Build history of the part. All positions in model axes, mm. A direction names the side the tool comes from. Round coordinates to 2 decimals unless told otherwise and drop trailing zeros. Write each loop counter-clockwise with the first axis right and the second up, starting at its lowest first coordinate (ties: lowest second). Pieces come first, ordered by that corner, then holes.
1) Saw through at A-A (z = 0). Write the cut outline in (x, y).
2) Saw through at B-B (x = 0). Write the cut outline in (y, z), plus the area to 3 significant figures.
3) Saw through at C-C (y = 11.25). Write the cut outline in (x, z).
4) Wall check: probe 1 along X at (y, z) = (25.75, -10.5); probe 2 along X at (y, z) = (26.05, 0); probe 3 along X at (y, z) = (13.75, -4). Give the ranges that are in metal, low to high.
5) Pull direction Z, two halves, no side cores. Call faces 3 (the cylindrical face through (24.986, 0.301, -14.715)), 4 (the cylindrical face through (-24.99, 14.58, 0.27)), 5 (the flat face through (24, 12, 0)): +Z half, -Z half, draft (parallel to the pull), parting line (faces both ways), or undercut.
6) Saw through at D-D (x = 20). Write the cut outline in (y, z), plus the area to 3 significant figures.
7) Which spindle directions (+Z, -Z, +X, -X, +Y, -Y) get a long thin tool onto all of the face, cutting with end or side? Do faces 1 (the cylindrical face through (24.986, 0.285, 6.501)), 2 (the flat face through (0, 26.8, 7)). Say none if no direction does.
8) Flat gauge pin, fed straight in: pin 1 (8 mm diameter, centred on x = 7.5, z = -9, fed in from -Y). Where does the tip first touch, or does it go through?
from build123d import *

# Parameters (mm, degrees)
BOSS_EXTRU_1_DEPTH      = 15
ESQUISSE4_R             = 6.25
ESQUISSE4_R_2           = 1.55
ENL_V_MAT_EXTRU_2_DEPTH = 41.239781312
ESQUISSE2_R             = 1.25
ENL_V_MAT_EXTRU_1_DEPTH = 61.392383626
CONG_1_R                = 1


with BuildPart() as part:
    # Esquisse1 → Boss.-Extru.1 (new, symmetric)
    with BuildSketch(Plane.XY):
        Polygon((-26, 26.8), (26, 26.8), (26, 0), (24, 0), (24, 24.8), (-24, 24.8), (-24, 0), (-26, 0), align=None)
    extrude(amount=BOSS_EXTRU_1_DEPTH, both=True)

    # Esquisse4 → Enlèv. mat.-Extru.2 (cut, through all)
    with BuildSketch(Plane(origin=(0, 26.8, 0), x_dir=(1, 0, 0), z_dir=(0, 1, 0))):
        with Locations(Location((0, 0, 0), (0, 0, 270))):
            Circle(ESQUISSE4_R)
        with Locations(Location((-8.485281374, 8.485281374, 0), (0, 0, 270))):
            Circle(ESQUISSE4_R_2)
        with Locations(Location((8.485281374, 8.485281374, 0), (0, 0, 270))):
            Circle(ESQUISSE4_R_2)
        with Locations(Location((8.485281374, -8.485281374, 0), (0, 0, 270))):
            Circle(ESQUISSE4_R_2)
        with Locations(Location((-8.485281374, -8.485281374, 0), (0, 0, 270))):
            Circle(ESQUISSE4_R_2)
        with Locations(Location((20, 10.5, 0), (0, 0, 270))):
            Circle(ESQUISSE4_R_2)
        with Locations(Location((-20, 10.5, 0), (0, 0, 270))):
            Circle(ESQUISSE4_R_2)
        with Locations(Location((20, -10.5, 0), (0, 0, 270))):
            Circle(ESQUISSE4_R_2)
        with Locations(Location((-20, -10.5, 0), (0, 0, 270))):
            Circle(ESQUISSE4_R_2)
    extrude(amount=-ENL_V_MAT_EXTRU_2_DEPTH, mode=Mode.SUBTRACT)

    # Esquisse2 → Enlèv. mat.-Extru.1 (cut, through all)
    with BuildSketch(Plane(origin=(26, 0, 0), x_dir=(0, 0, -1), z_dir=(1, 0, 0))):
        with Locations((-12, 15.8)):
            Circle(ESQUISSE2_R)
        with Locations((-12, 3.8)):
            Circle(ESQUISSE2_R)
        with Locations((0, 15.8)):
            Circle(ESQUISSE2_R)
        with Locations((12, 3.8)):
            Circle(ESQUISSE2_R)
        with Locations((12, 15.8)):
            Circle(ESQUISSE2_R)
        with BuildLine():
            Line((-6.2, 3.8), (-6.2, 0))
            Line((-6.2, 0), (6.2, 0))
            Line((6.2, 0), (6.2, 3.8))
            ThreePointArc((6.2, 3.8), (0, 10), (-6.2, 3.8))
        make_face()
    extrude(amount=-ENL_V_MAT_EXTRU_1_DEPTH, mode=Mode.SUBTRACT)

    # Congé1
    cong_1_edges = [part.edges().sort_by_distance(p)[0] for p in [
        (-25, 0, -6.2),
        (25, 0, -6.2),
        (-25, 0, 6.2),
        (25, 0, 6.2),
        (25, 0, 15),
        (-25, 0, 15),
        (-25, 0, -15),
        (25, 0, -15),
    ]]
    fillet(cong_1_edges, radius=CONG_1_R)


solid = part.part
Evaluation:
1. outline: (-26, 10) - (-24, 10) - (-24, 14.55) - (-26, 14.55) - close; (-26, 17.05) - (-24, 17.05) - (-24, 24.8) - (-6.25, 24.8) - (-6.25, 26.8) - (-26, 26.8) - close; (6.25, 24.8) - (24, 24.8) - (24, 17.05) - (26, 17.05) - (26, 26.8) - (6.25, 26.8) - close; (24, 10) - (26, 10) - (26, 14.55) - (24, 14.55) - close
2. outline: (24.8, -15) - (26.8, -15) - (26.8, -6.25) - (24.8, -6.25) - close; (24.8, 6.25) - (26.8, 6.25) - (26.8, 15) - (24.8, 15) - close
2. area: 35.0 mm2
3. outline: (-26, -15) - (-24, -15) - (-24, 15) - (-26, 15) - close; (24, -15) - (26, -15) - (26, 15) - (24, 15) - close
4. probe 1: x = -26 to -21.55, -18.45 to 18.45, 21.55 to 26
4. probe 2: x = -26 to -6.25, 6.25 to 26
4. probe 3: x = -26 to -24, 24 to 26
5. face 3: -Z half
5. face 4: undercut
5. face 5: draft
6. outline: (24.8, -15) - (26.8, -15) - (26.8, -12.05) - (24.8, -12.05) - close; (24.8, -8.95) - (26.8, -8.95) - (26.8, 8.95) - (24.8, 8.95) - close; (24.8, 12.05) - (26.8, 12.05) - (26.8, 15) - (24.8, 15) - close
6. area: 47.6 mm2
7. face 1: +X, -X, -Y
7. face 2: +Z, -Z, +X, -X, +Y
8. pin 1: stops at y = 24.8
